Verification items for this drawing (mm, ordinates from the low corner). A direction names the side the tool comes from. Round coordinates to 2 decimals unless told otherwise and drop trailing zeros. Loops run counter-clockwise (first coordinate to the right, second up) from the corner with the lowest first, then second, coordinate; pieces in that order, holes last. Notation, with made-up numbers: M -5,-27 L 7,-27 A3 ccw 7,-23 Z; hole C 72.5,26.25 d8. An arc over 180 degrees is marked long. Write item = value, one per line.
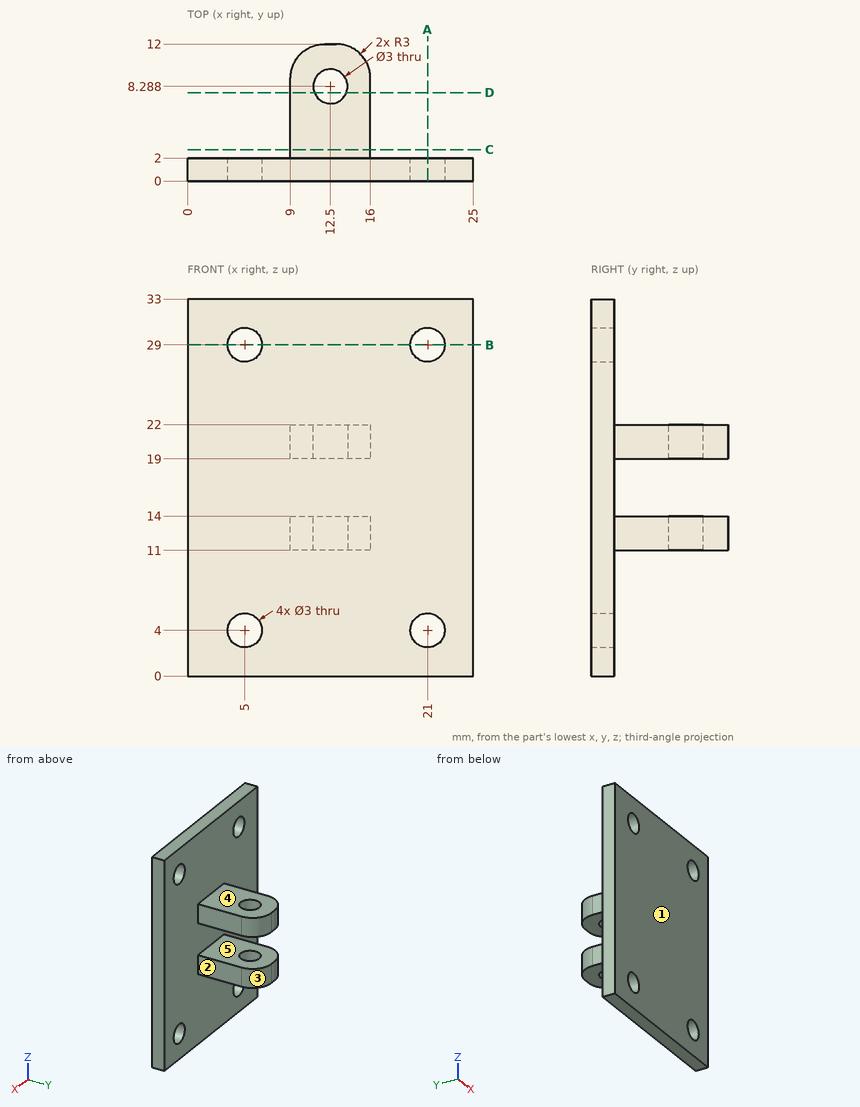
(1) Sectioned sample at A-A on x = 21. Record the cut outline in (y, z).
Result set:
outline = M 0,0 L 2,0 L 2,2.5 L 0,2.5 Z; M 0,5.5 L 2,5.5 L 2,27.5 L 0,27.5 Z; M 0,30.5 L 2,30.5 L 2,33 L 0,33 Z
(2) Sectioned sample at B-B on z = 29. Record the cut outline in (x, y).
Result set:
outline = M 0,0 L 3.5,0 L 3.5,2 L 0,2 Z; M 6.5,0 L 19.5,0 L 19.5,2 L 6.5,2 Z; M 22.5,0 L 25,0 L 25,2 L 22.5,2 Z
(3) Sectioned sample at D-D on y = 7.75. Record the cut outline in (x, z).
Result set:
outline = M 9,11 L 11.1,11 L 11.1,14 L 9,14 Z; M 9,19 L 11.1,19 L 11.1,22 L 9,22 Z; M 13.9,11 L 16,11 L 16,14 L 13.9,14 Z; M 13.9,19 L 16,19 L 16,22 L 13.9,22 Z
(4) Tool access check on the marked faces 1 and 2. Record the directions out of +Z, -Z, +X, -X, +Y, -Y that give a thin tool (end or side, any length) a straight path to the whole face; none if there is none.
Result set:
face_1 = +Z, -Z, +X, -X, -Y
face_2 = +Z, -Z, +X, +Y
(5) Release check for a two-part mould opening along Z. For the marked faces 3, 4 and 5 record: released by +Z, released by -Z, zero draft, split by the parting line, or undercut.
Result set:
face_3 = zero draft
face_4 = released by +Z
face_5 = undercut
(6) Material ranges on line 1 along X through (y, z) = (1.4, 29); line 2 along Z through (x, y) = (5, 0.5); line 3 along Z through (x, y) = (14.25, 4.5), recorded low to high. Write a range as from..to.
Result set:
line_1 = 0..3.5, 6.5..19.5, 22.5..25
line_2 = 0..2.5, 5.5..27.5, 30.5..33
line_3 = 11..14, 19..22
(7) Depth check by flat-ended pin: pin 1 Ø5 at (x, z) = (20.5, 29.5) entering from +Y; pin 2 Ø1.5 at (y, z) = (7, 12.5) entering from -X; pin 3 Ø5 at (y, z) = (7.5, 9) entering from +X; pin 4 Ø2.5 at (x, y) = (12.5, 8.29) entering from +Z. Enter the tip coordinate at first touch or a pass-through.
Result set:
pin_1 = 2
pin_2 = 9
pin_3 = 16
pin_4 = through
(8) Sectioned sample at C-C on y = 2.75. Record the cut outline in (x, z).
Result set:
outline = M 9,11 L 16,11 L 16,14 L 9,14 Z; M 9,19 L 16,19 L 16,22 L 9,22 Z
